Part print with two shaded views. Sizes in mm from the minimum x, y, z corner. Round coordinates to 2 decimals unless told otherwise and drop trailing zeros. Order: outer loops, then holes, each group sorted by start corner. A loop starts at its lowest first (then second) coordinate and runs counter-clockwise, first axis right, second up. Notation, with made-up numbers: (-22, 31.5) - (-11, 31.5) arc R12 ccw to (-11, 53.5) - close; hole circle Ø2 at (79.5, -21.75). An arc over 180 degrees is marked (long way). Answer as CSV lines item,"result". Start each with the question number.
1. Band-saw the part on B-B on z = 1.75. List the corners of the cut face in (x, y).
2. Pull direction Z, two halves, no side cores. Call the marked faces 1, 2 and 3: released by +Z, released by -Z, zero draft, split by the parting line, or undercut.
3. Wall check: line 1 along Z through (x, y) = (1.3, 3); line 2 along Z through (x, y) = (0.8, 3.5) (1 decimal); line 3 along Z through (x, y) = (1.25, 1.5). Give the ranges that are in metal, low to high. Write a range as [from, to].
4. Band-saw the part on A-A on x = 0.25. List the corners of the cut face in (y, z), then the cut area to 3 significant figures.
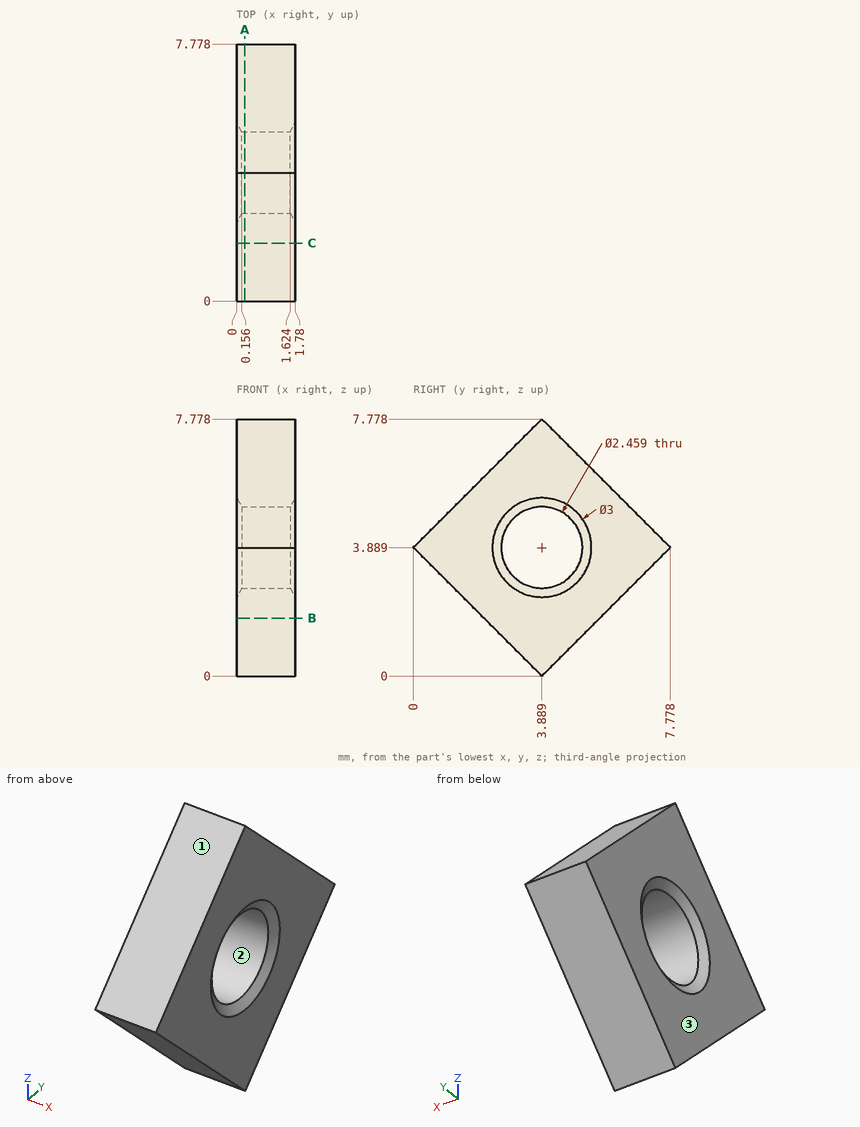
Reply:
1,outline,"(0, 2.14) - (1.78, 2.14) - (1.78, 5.64) - (0, 5.64) - close"
2,face 1,"released by +Z"
2,face 2,"undercut"
2,face 3,"zero draft"
3,line 1,"z = [0.89, 3.04], [4.74, 6.89]"
3,line 2,"z = [0.4, 2.7], [5.1, 7.4]"
3,line 3,"z = [2.39, 5.39]"
4,outline,"(0, 3.89) - (3.89, 0) - (7.78, 3.89) - (3.89, 7.78) - close; hole circle Ø2.46 at (3.89, 3.89)"
4,area,"25.5 mm2"
